Geometry: final body of the model. Coordinates: model frame, mm. Face numbers are marked on the shaded views. A direction names the side the tool comes from. Coordinates: 2 decimals unless noted, no trailing zeros. Order: outer loops, then holes, each group sorted by start corner. A loop starts at its lowest first (then second) coordinate and runs counter-clockwise, first axis right, second up. Notation, with made-up numbers: (-14, 78) -> (1, 78) arc R8 cw to (1, 89) -> close; hole circle Ø10 at (-8.5, 52). An arc over 180 degrees is marked (long way). Answer in a Markdown table with one row per item. Add a question column.
1) Section query D-D on y = 78. Return the cut outline in (x, z), then the cut area to 3 significant figures.
2) Section query A-A on y = 16. Return the cut outline in (x, z), then the cut area to 3 significant figures.
3) Set-up query: the marked faces 1 and 2. Return all of +Z, -Z, +X, -X, +Y, -Y with unobstructed straight access to the full face (end or side cutting, diameter ignored); none if empty.
4) Contact query for flat-ended pins moving along their axis: P1, Ø2, axis at x = 106, z = 85.5, coming from the +Y side; P2, Ø8, axis at y = 97, z = 225, coming from the +X side; P3, Ø12, axis at y = 16.5, z = 59, coming from the +X side; P4, Ø1, axis at x = 25, z = 211.5, coming from the -Y side. Output: stop coordinate, or through.
5) Section query B-B on x = 75. Return the cut outline in (y, z) (1 decimal).
6) Pull-direction query (Y, two-part tool) for the marked faces 3, 4 and 5; classes: +Y half, -Y half, draft (parallel to the pull), parting line (faces both ways), or undercut.
7) Section query C-C on z = 260. Return the cut outline in (x, y).
8) Ray query, line 1 (X direction, y = 18, z = 46); line 2 (Y direction, x = 13.5, z = 266.5); line 3 (Y direction, x = 107, z = 154). Return the intervals inside material, ascending. Write a range as from..to.
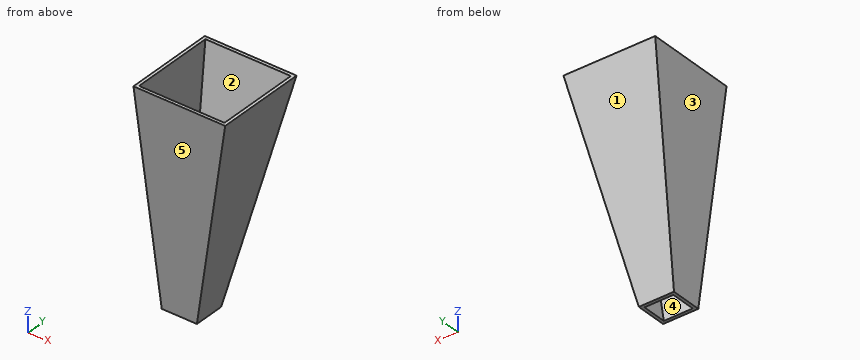
```python
from build123d import *

# Parameters (mm, degrees)
SKETCH1_W           = 140.843
SKETCH1_H           = 139.954
BOSS_EXTRUDE1_DEPTH = 304.8
CUT_EXTRUDE1_DEPTH  = 364.767663166
CUT_EXTRUDE2_DEPTH  = 364.767663166
SHELL1_T            = -4.7625


with BuildPart() as part:
    # Sketch1 → Boss-Extrude1 (new body)
    with BuildSketch(Plane.XY):
        with Locations((70.4215, 69.977)):
            Rectangle(SKETCH1_W, SKETCH1_H)
    extrude(amount=BOSS_EXTRUDE1_DEPTH)

    # Sketch2 → Cut-Extrude1 (cut, through all)
    with BuildSketch(Plane(origin=(140.843, 0, 0), x_dir=(0, 0, -1), z_dir=(1, 0, 0))):
        Polygon((-304.8, 139.954), (0, 47.625), (0, 139.954), align=None)
    extrude(amount=-CUT_EXTRUDE1_DEPTH, mode=Mode.SUBTRACT)

    # Sketch3 → Cut-Extrude2 (cut, through all)
    with BuildSketch(Plane.XZ):
        Polygon((140.843, 304.8), (97.4344, 0), (140.843, 0), align=None)
        Polygon((0, 304.8), (43.4086, 0), (0, 0), align=None)
    extrude(amount=-CUT_EXTRUDE2_DEPTH, mode=Mode.SUBTRACT)

    # Shell1
    shell1_openings = [part.faces().sort_by_distance(p)[0] for p in [
        (70.4215, 69.977, 304.8),
        (70.4215, 23.8125, 0),
    ]]
    offset(amount=SHELL1_T, openings=shell1_openings, kind=Kind.INTERSECTION)


solid = part.part
```
Result:
| question | item | result |
|---|---|---|
| 1 | outline | (0, 304.8) -> (29.13, 100.28) -> (111.72, 100.28) -> (140.84, 304.8) -> (136.03, 304.8) -> (109.24, 116.7) -> (31.6, 116.7) -> (4.81, 304.8) -> close |
| 1 | area | 3,200 mm2 |
| 2 | outline | (0, 304.8) -> (43.41, 0) -> (48.22, 0) -> (4.81, 304.8) -> close; (92.62, 0) -> (97.43, 0) -> (140.84, 304.8) -> (136.03, 304.8) -> close |
| 2 | area | 2,930 mm2 |
| 3 | face 1 | -Z, +X, -X, +Y |
| 3 | face 2 | +Z |
| 4 | P1 | y = 73.83 |
| 4 | P2 | x = 130.05 |
| 4 | P3 | x = 106.69 |
| 4 | P4 | y = 0 |
| 5 | outline | (0, 0) -> (4.8, 0) -> (4.8, 304.8) -> (0, 304.8) -> close; (42.6, 0) -> (47.6, 0) -> (140, 304.8) -> (135, 304.8) -> close |
| 6 | face 3 | draft |
| 6 | face 4 | undercut |
| 6 | face 5 | -Y half |
| 7 | outline | (6.38, 0) -> (134.46, 0) -> (134.46, 126.38) -> (6.38, 126.38) -> close; hole (11.19, 4.76) -> (129.65, 4.76) -> (129.65, 121.41) -> (11.19, 121.41) -> close |
| 8 | line 1 | 36.86..41.67, 99.18..103.99 |
| 8 | line 2 | 0..4.76, 123.38..128.35 |
| 8 | line 3 | 0..4.76, 89.3..94.27 |
